Model file for the job. Use its own axes, mm. Face numbers are marked on the shaded views. A direction names the side the tool comes from. Coordinates: 2 decimals unless noted, no trailing zeros. Order: outer loops, then holes, each group sorted by start corner. A loop starts at its lowest first (then second) coordinate and runs counter-clockwise, first axis right, second up. Notation, with made-up numbers: (33.25, 66.25) -> (56.25, 66.25) arc R14 cw to (56.25, 85.25) -> close; hole circle Ø9 at (87.5, 49.5). An arc over 180 degrees is marked (long way). Return JSON: item names as keys, results as strings. Group by question number.
1) Cut at D-D (y = -111). Write the cut outline in (x, z), and give its area (3 significant figures).
2) Cut at C-C (y = -72.5). Write the cut outline in (x, z).
3) Cut at A-A (y = -96.52). Write the cut outline in (x, z).
4) Flat gauge pins, fed straight in: pin 1 (14 mm diameter, centred on x = 18, y = -83, fed in from -Z); pin 2 (24.5 mm diameter, centred on x = 48.08, z = -14.13, fed in from -Y). Where does each tip first touch, or does it go through?
5) Probe line 1 (X direction, y = -118, z = 40); line 2 (Y direction, x = 5, z = -28); line 3 (Y direction, x = -51.5, z = -8). List the from-to ranges inside material, lowest first.
6) Pull direction Z, two halves, no side cores. Call the marked faces 1, 2 and 3: +Z half, -Z half, draft (parallel to the pull), parting line (faces both ways), or undercut.
7) Cut at B-B (y = -18). Write the cut outline in (x, z), and give its area (3 significant figures).
8) Which spindle directions (+Z, -Z, +X, -X, +Y, -Y) get a long thin tool onto all of the face, cutting with end or side? Do the marked faces 4, 5 and 6. Say none if no direction does.
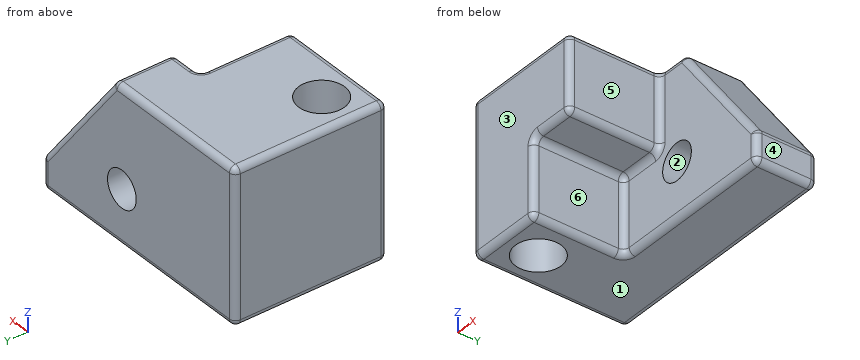
from build123d import *

# Parameters (mm, degrees)
F0_W      = 203.2
F0_H      = 127
F1_DEPTH  = 127
F3_DEPTH  = 76.2
F4_SIZE2  = 101.6
F4_SIZE   = 76.2
F5_R      = 5.08
F7_R      = 15.24
F8_DEPTH  = 50.8
F9_R      = 19.05
F10_DEPTH = 127


# Not quite as in the source:
# - a feature of the source that left no trace in its solid (it failed there, or was rolled back) is left out


with BuildPart() as f1:
    # F0 (on Front) → F1 (new body)
    with BuildSketch(Plane.XZ):
        with Locations((30.3024339037, 3.653427586)):
            Rectangle(F0_W, F0_H)
    extrude(amount=F1_DEPTH)

    # F2 (on face) → F3 (cut)
    with BuildSketch(Plane.XZ.offset(127)):
        Polygon((-7.7975660963, 3.653427586), (-7.7975660963, -59.846572414), (131.9024339037, -59.846572414), (131.9024339037, 67.153427586), (30.3024339037, 67.153427586), (30.3024339037, 3.653427586), align=None)
    extrude(amount=-F3_DEPTH, mode=Mode.SUBTRACT)

    # F4
    f4_edges = [f1.edges().sort_by_distance(p)[0] for p in [
        (131.902434, -25.4, 67.153428),
    ]]
    f4_side = f1.faces().sort_by_distance((8.531005, -52.614286, 67.153428))[0]
    chamfer(f4_edges, length=F4_SIZE, length2=F4_SIZE2, reference=f4_side)

    # F5
    f5_edges = [f1.edges().sort_by_distance(p)[0] for p in [
        (30.302434, -88.9, 67.153428),
        (-20.497566, -127, 67.153428),
        (55.702434, -25.4, 67.153428),
        (131.902434, -25.4, -34.446572),
        (131.902434, -25.4, -59.846572),
        (-39.547566, -127, -59.846572),
        (-7.797566, -88.9, -59.846572),
        (-7.797566, -127, -28.096572),
        (30.302434, -88.9, 3.653428),
        (30.302434, -127, 35.403428),
        (30.302434, -50.8, 35.403428),
        (11.252434, -50.8, 3.653428),
        (-7.797566, -50.8, -28.096572),
        (93.802434, 0, 16.353428),
        (131.902434, 0, -47.146572),
        (-7.797566, 0, 67.153428),
        (30.302434, 0, -59.846572),
        (-71.297566, 0, 3.653428),
        (-71.297566, -63.5, 67.153428),
        (-71.297566, -63.5, -59.846572),
        (131.902434, -50.8, -47.146572),
        (93.802434, -50.8, 16.353428),
        (62.052434, -50.8, -59.846572),
        (43.002434, -50.8, 67.153428),
        (-71.297566, -127, 3.653428),
        (-7.797566, -88.9, 3.653428),
        (11.252434, -127, 3.653428),
    ]]
    fillet(f5_edges, radius=F5_R)

    # F7 (on face) → F8 (cut, through all)
    with BuildSketch(Plane.XZ.offset(50.8)):
        with Locations((48.0824339037, -14.126572414)):
            Circle(F7_R)
    extrude(amount=-F8_DEPTH, mode=Mode.SUBTRACT)

    # F9 (on face) → F10 (cut, through all)
    with BuildSketch(Plane.XY.offset(67.153427586)):
        with Locations((-40.8175660963, -96.52)):
            Circle(F9_R)
    extrude(amount=-F10_DEPTH, mode=Mode.SUBTRACT)


solid = f1.part
Answers below:
{
 "1": {"outline": "(-71.3, -54.77) arc R5.08 ccw to (-66.22, -59.85) -> (-53.2, -59.85) -> (-53.2, 67.15) -> (-66.22, 67.15) arc R5.08 ccw to (-71.3, 62.07) -> close; (-28.44, -59.85) -> (-12.88, -59.85) arc R5.08 ccw to (-7.8, -54.77) -> (-7.8, -1.43) arc R5.08 cw to (-2.72, 3.65) -> (25.22, 3.65) arc R5.08 ccw to (30.3, 8.73) -> (30.3, 62.07) arc R5.08 ccw to (25.22, 67.15) -> (-28.44, 67.15) -> close", "area": "7,320 mm^2"},
 "2": {"outline": "(-71.3, -54.77) arc R5.08 ccw to (-66.22, -59.85) -> (-12.88, -59.85) arc R5.08 ccw to (-7.8, -54.77) -> (-7.8, -1.43) arc R5.08 cw to (-2.72, 3.65) -> (25.22, 3.65) arc R5.08 ccw to (30.3, 8.73) -> (30.3, 62.07) arc R5.08 ccw to (25.22, 67.15) -> (-66.22, 67.15) arc R5.08 ccw to (-71.3, 62.07) -> close"},
 "3": {"outline": "(-71.3, -54.77) arc R5.08 ccw to (-66.22, -59.85) -> (-59.87, -59.85) -> (-59.87, 67.15) -> (-66.22, 67.15) arc R5.08 ccw to (-71.3, 62.07) -> close; (-21.77, -59.85) -> (-12.88, -59.85) arc R5.08 ccw to (-7.8, -54.77) -> (-7.8, -1.43) arc R5.08 cw to (-2.72, 3.65) -> (25.22, 3.65) arc R5.08 ccw to (30.3, 8.73) -> (30.3, 62.07) arc R5.08 ccw to (25.22, 67.15) -> (-21.77, 67.15) -> close"},
 "4": {"pin 1": "stops at z = 3.65", "pin 2": "passes through"},
 "5": {"line 1": "x = -71.3 to 30.3", "line 2": "y = -50.8 to 0", "line 3": "y = -127 to -112.29, -80.75 to 0"},
 "6": {"face 1": "-Z half", "face 2": "undercut", "face 3": "draft"},
 "7": {"outline": "(-71.3, -54.77) arc R5.08 ccw to (-66.22, -59.85) -> (126.82, -59.85) arc R5.08 ccw to (131.9, -54.77) -> (131.9, -36.14) arc R5.08 ccw to (130.89, -33.09) -> (57.23, 65.12) arc R5.08 ccw to (53.16, 67.15) -> (-66.22, 67.15) arc R5.08 ccw to (-71.3, 62.07) -> close; hole circle Ø30.48 at (48.08, -14.13)", "area": "21,200 mm^2"},
 "8": {"face 4": "+Z, -Z, +X, +Y, -Y", "face 5": "+Z, -Z, +X, -Y", "face 6": "-Z, +X, -Y"}
}
